```python
from build123d import *

# Parameters (mm, degrees)
SKETCH1_W           = 130
SKETCH1_H           = 100
BOSS_EXTRUDE1_DEPTH = 5
SKETCH2_W           = 10
SKETCH2_H           = 10
BOSS_EXTRUDE2_DEPTH = 160
SKETCH3_W           = 10
SKETCH3_H           = 10
BOSS_EXTRUDE3_DEPTH = 110
SKETCH4_W           = 10
SKETCH4_H           = 10
BOSS_EXTRUDE4_DEPTH = 110
SKETCH5_W           = 10
SKETCH5_H           = 10
BOSS_EXTRUDE5_DEPTH = 80
SKETCH6_W           = 10
SKETCH6_H           = 10
BOSS_EXTRUDE6_DEPTH = 80
SKETCH9_W           = 9
SKETCH9_H           = 8
CUT_EXTRUDE4_DEPTH  = 163


with BuildPart() as part:
    # Sketch1 → Boss-Extrude1 (new body)
    with BuildSketch(Plane.XY):
        with Locations((65, 50)):
            Rectangle(SKETCH1_W, SKETCH1_H)
    extrude(amount=BOSS_EXTRUDE1_DEPTH)

    # Sketch2 → Boss-Extrude2 (add)
    with BuildSketch(Plane.XY.offset(5)):
        with Locations((5, 95)):
            Rectangle(SKETCH2_W, SKETCH2_H)
        with Locations((125, 95)):
            Rectangle(SKETCH2_W, SKETCH2_H)
        with Locations((5, 5)):
            Rectangle(SKETCH2_W, SKETCH2_H)
        with Locations((125, 5)):
            Rectangle(SKETCH2_W, SKETCH2_H)
    extrude(amount=BOSS_EXTRUDE2_DEPTH)

    # Sketch3 → Boss-Extrude3 (add)
    with BuildSketch(Plane(origin=(10, 0, 0), x_dir=(0, 0, -1), z_dir=(1, 0, 0))):
        with Locations((-160, 5)):
            Rectangle(SKETCH3_W, SKETCH3_H)
    extrude(amount=BOSS_EXTRUDE3_DEPTH)

    # Sketch4 → Boss-Extrude4 (add)
    with BuildSketch(Plane(origin=(10, 0, 0), x_dir=(0, 0, -1), z_dir=(1, 0, 0))):
        with Locations((-160, 95)):
            Rectangle(SKETCH4_W, SKETCH4_H)
    extrude(amount=BOSS_EXTRUDE4_DEPTH)

    # Sketch5 → Boss-Extrude5 (add)
    with BuildSketch(Plane.XZ.offset(-90)):
        with Locations((5, 160)):
            Rectangle(SKETCH5_W, SKETCH5_H)
    extrude(amount=BOSS_EXTRUDE5_DEPTH)

    # Sketch6 → Boss-Extrude6 (add)
    with BuildSketch(Plane.XZ.offset(-90)):
        with Locations((125, 160)):
            Rectangle(SKETCH6_W, SKETCH6_H)
    extrude(amount=BOSS_EXTRUDE6_DEPTH)

    # Sketch9 → Cut-Extrude4 (cut)
    with BuildSketch(Plane.XY.offset(165)):
        with Locations((124.5, 94.920029207)):
            Rectangle(SKETCH9_W, SKETCH9_H)
        with Locations((124.5, 5)):
            Rectangle(SKETCH9_W, SKETCH9_H)
        with Locations((5.5, 5.741486023)):
            Rectangle(SKETCH9_W, SKETCH9_H)
        with Locations((5.995524186, 95)):
            Rectangle(SKETCH9_W, SKETCH9_H)
    extrude(amount=-CUT_EXTRUDE4_DEPTH, mode=Mode.SUBTRACT)


solid = part.part
```
The listing builds one solid part. Answer for the finished solid, in the listing's coordinates (mm). A direction names the side the tool comes from. Round coordinates to 2 decimals unless told otherwise and drop trailing zeros. Loops run counter-clockwise (first coordinate to the right, second up) from the corner with the lowest first, then second, coordinate; pieces in that order, holes last.
1) Consider line 1 (Y direction, x = 124, z = 55); line 2 (X direction, y = 75.5, z = 156); line 3 (Z direction, x = 8, y = 64). Determine where each line is inside the solid, lowest interval first.
Outcome:
line 1: y = 0 to 1, 9 to 10, 90 to 90.92, 98.92 to 100
line 2: x = 0 to 10, 120 to 130
line 3: z = 0 to 5, 155 to 165
2) A cutting plane is placed at A-A on z = 118.5. Give the number of separate pieces and of enclosed holes in the cut face, plus the area to 3 significant figures.
Outcome:
separate pieces: 4
enclosed holes: 0
area: 116 mm2
3) A cutting plane is placed at B-B on y = 18. Determine the outline of the cut face in (x, z).
Outcome:
outline: (0, 0) - (130, 0) - (130, 5) - (0, 5) - close; (0, 155) - (10, 155) - (10, 165) - (0, 165) - close; (120, 155) - (130, 155) - (130, 165) - (120, 165) - close
4) Given P1, Ø2.5, axis at x = 124.5, y = 94.5, coming from the +Z side; P2, Ø4, axis at x = 106.5, y = 37, coming from the +Z side, each flat-ended and moving along its own axis, determine where each tip first touches the part or whether it passes through.
Outcome:
P1: stops at z = 2
P2: stops at z = 5
5) A cutting plane is placed at C-C on x = 109. Determine the outline of the cut face in (y, z), plus the area to 3 significant figures.
Outcome:
outline: (0, 0) - (100, 0) - (100, 5) - (0, 5) - close; (0, 155) - (10, 155) - (10, 165) - (0, 165) - close; (90, 155) - (100, 155) - (100, 165) - (90, 165) - close
area: 700 mm2
6) For a pull along Y with two mould halves and no side action, classify faces 1 (the face through (10, 6, 160)), 2 (the face through (0, 91, 88)), 3 (the face through (122, 0, 101)) as released by +Y, released by -Y, zero draft, split by the parting line, or undercut.
Outcome:
face 1: undercut
face 2: zero draft
face 3: released by -Y
7) For faces 4 (the face through (124, 95, 2)), 5 (the face through (125, 51, 155)), 6 (the face through (64, 51, 5)), determine the directions among +Z, -Z, +X, -X, +Y, -Y from which every point of the face is accessible in a straight line to the end or side of a thin tool.
Outcome:
face 4: +Z
face 5: +X, -X
face 6: none
